from build123d import *

# Parameters (mm, degrees)
SKETCH1_W           = 72.5
SKETCH1_H           = 75
BOSS_EXTRUDE1_DEPTH = 5
SKETCH2_R           = 27.1
SKETCH2_R_2         = 25.1
BOSS_EXTRUDE2_DEPTH = 5
SKETCH4_W           = 2.7
SKETCH4_H           = 75
BOSS_EXTRUDE3_DEPTH = 5.6
SKETCH5_R           = 0.5
BOSS_EXTRUDE4_DEPTH = 75
SKETCH6_W           = 0.9
SKETCH6_H           = 10.6
CUT_EXTRUDE1_DEPTH  = 84.972748556
FILLET1_R           = 2
FILLET2_R           = 1
FILLET3_R           = 1.5
FILLET4_R           = 1.5
SKETCH3_R           = 0.5


with BuildPart() as part:
    # Sketch1 → Boss-Extrude1 (new body)
    with BuildSketch(Plane(origin=(0, 0, 0), x_dir=(1, 0, 0), z_dir=(0, 1, 0))):
        Rectangle(SKETCH1_W, SKETCH1_H)
    extrude(amount=BOSS_EXTRUDE1_DEPTH)

    # Sketch2 → Boss-Extrude2 (add)
    with BuildSketch(Plane.XZ):
        with Locations(Location((0, 0, 0), (0, 0, 90))):
            Circle(SKETCH2_R)
        with Locations(Location((0, 0, 0), (0, 0, 270))):
            Circle(SKETCH2_R_2, mode=Mode.SUBTRACT)
    extrude(amount=BOSS_EXTRUDE2_DEPTH)

    # Sketch4 → Boss-Extrude3 (add)
    with BuildSketch(Plane(origin=(0, 5, 0), x_dir=(1, 0, 0), z_dir=(0, 1, 0))):
        with Locations((-34.9, 0)):
            Rectangle(SKETCH4_W, SKETCH4_H)
        with Locations((34.9, 0)):
            Rectangle(SKETCH4_W, SKETCH4_H)
    extrude(amount=BOSS_EXTRUDE3_DEPTH)

    # Sketch5 → Boss-Extrude4 (add)
    with BuildSketch(Plane.XY.offset(37.5)):
        with Locations((-33.55, 10.1)):
            Circle(SKETCH5_R)
        with Locations((33.55, 10.1)):
            Circle(SKETCH5_R)
    extrude(amount=-BOSS_EXTRUDE4_DEPTH)

    # Sketch6 → Cut-Extrude1 (cut, through all)
    with BuildSketch(Plane(origin=(0, 0, -37.5), x_dir=(-1, 0, 0), z_dir=(0, 0, -1))):
        with Locations((-35.8, 5.3)):
            Rectangle(SKETCH6_W, SKETCH6_H)
        with Locations((35.8, 5.3)):
            Rectangle(SKETCH6_W, SKETCH6_H)
    extrude(amount=-CUT_EXTRUDE1_DEPTH, mode=Mode.SUBTRACT)

    # Fillet1
    fillet1_edges = [part.edges().sort_by_distance(p)[0] for p in [
        (0, 0, -27.1),
    ]]
    fillet(fillet1_edges, radius=FILLET1_R)

    # Fillet2
    fillet2_edges = [part.edges().sort_by_distance(p)[0] for p in [
        (0, -5, 25.1),
    ]]
    fillet(fillet2_edges, radius=FILLET2_R)

    # Fillet3
    fillet3_edges = [part.edges().sort_by_distance(p)[0] for p in [
        (0, 0, -37.5),
        (0, 0, 37.5),
        (35.35, 0, 0),
        (-35.35, 0, 0),
    ]]
    fillet(fillet3_edges, radius=FILLET3_R)

    # Fillet4
    fillet4_edges = [part.edges().sort_by_distance(p)[0] for p in [
        (35.35, 10.6, 0),
        (-35.35, 10.6, 0),
    ]]
    fillet(fillet4_edges, radius=FILLET4_R)

    # Sketch3 → Revolve1 (revolve)
    with BuildSketch(Plane(origin=(0, 0, 0), x_dir=(0, 0, -1), z_dir=(1, 0, 0))):
        with Locations((-25.05, -1)):
            Circle(SKETCH3_R)
    revolve(axis=Axis((0, 0, 0), (0, -1, 0)))


solid = part.part
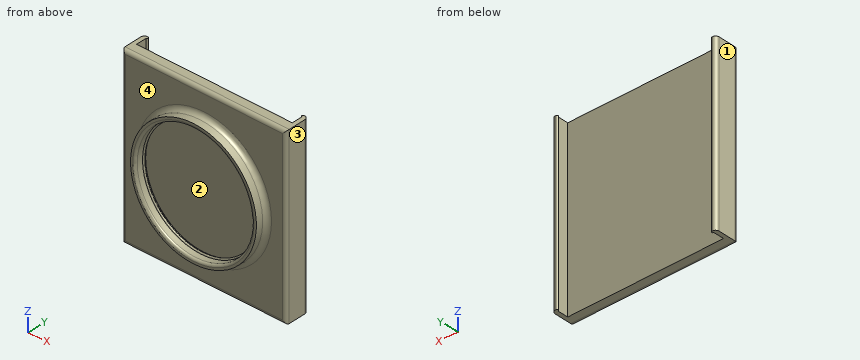
Design review of the part built by this model. Coordinates are the model's own, in mm. Face numbers are marked on the shaded views. A direction names the side the tool comes from. Coordinates: 2 decimals unless noted, no trailing zeros. Loops run counter-clockwise (first coordinate to the right, second up) from the corner with the lowest first, then second, coordinate; pieces in that order, holes last. Notation, with made-up numbers: (70.25, 35.5) -> (91.25, 35.5) arc R30 ccw to (91.25, 71.5) -> close; hole circle Ø10 at (45.5, 59). An arc over 180 degrees is marked (long way). Use a Markdown table: item, result. Add a question column.
Item 1: Machinability: for the marked faces 3 and 4, which of the approach directions +Z, -Z, +X, -X, +Y, -Y give a long, thin tool a straight path to every point of the face, cutting with its end or side? Answer none if there is none.
Item 2: Clearance check with flat-ended pins moving along their axes: P1, Ø1, axis at x = 11, y = 7, coming from the -Z side; P2, Ø3, axis at x = 2, z = -9, coming from the -Y side; P3, Ø8, axis at x = 17, z = -14, coming from the +Y side. State where each tip first meets the part, or that it passes through.
Item 3: We need section C-C, the plane x = 0. Write out the cut boundary in (y, z).
Item 4: Wall thickness on L1, parallel to X at y = -3.15, z = 0; L2, parallel to Y at x = -17.5, z = -29.5; L3, parallel to X at y = -0.2, z = 0: over which ranges is each line inside the solid? List them lowest first. Write a range as from..to.
Item 5: The part is to be moulded in two halves that separate along Z. For the marked faces 1 and 2, say which applies: +Z half, -Z half, draft (parallel to the pull), parting line (faces both ways), or undercut.
Item 6: We need section A-A, the plane y = 7. Write out the cut boundary in (x, z).
Item 7: We need section B-B, the plane z = 31.5. Write out the cut boundary in (x, y), and give its area (3 significant figures).
Numbers:
| question | item | result |
|---|---|---|
| 1 | face 3 | +Z, -Z, +X, +Y, -Y |
| 1 | face 4 | -Y |
| 2 | P1 | passes through |
| 2 | P2 | stops at y = 0 |
| 2 | P3 | stops at y = 5 |
| 3 | outline | (-5, -27.1) -> (-2, -27.1) arc R2 cw to (0, -29.1) -> (0, -36) arc R1.5 ccw to (1.5, -37.5) -> (5, -37.5) -> (5, 37.5) -> (1.5, 37.5) arc R1.5 ccw to (0, 36) -> (0, 29.1) arc R2 cw to (-2, 27.1) -> (-5, 27.1) -> (-5, 26.1) arc R1 ccw to (-4, 25.1) -> (-1.5, 25.1) arc R0.5 ccw (long way) to (-0.5, 25.1) -> (0, 25.1) -> (0, -25.1) -> (-0.5, -25.1) arc R0.5 ccw (long way) to (-1.5, -25.1) -> (-4, -25.1) arc R1 ccw to (-5, -26.1) -> close |
| 4 | L1 | x = -27.1..-25.1, 25.1..27.1 |
| 4 | L2 | y = 0..5 |
| 4 | L3 | x = -28.23..-25.1, 25.1..28.23 |
| 5 | face 1 | draft |
| 5 | face 2 | undercut |
| 6 | outline | (-35.35, -37.5) -> (-33.55, -37.5) -> (-33.55, 37.5) -> (-35.35, 37.5) -> close; (33.55, -37.5) -> (35.35, -37.5) -> (35.35, 37.5) -> (33.55, 37.5) -> close |
| 7 | outline | (-35.35, 1.5) arc R1.5 ccw to (-33.85, 0) -> (33.85, 0) arc R1.5 ccw to (35.35, 1.5) -> (35.35, 9.1) arc R1.5 ccw to (33.85, 10.6) -> (33.55, 10.6) arc R0.5 ccw to (33.55, 9.6) -> (33.55, 5) -> (-33.55, 5) -> (-33.55, 9.6) arc R0.5 ccw to (-33.55, 10.6) -> (-33.85, 10.6) arc R1.5 ccw to (-35.35, 9.1) -> close |
| 7 | area | 373 mm^2 |
